Design review of the part built by this model. Coordinates are the model's own, in mm. A direction names the side the tool comes from. Give positions to 0.01 mm unless a question says otherwise; leave off trailing zeros. Order: outer loops, then holes, each group sorted by start corner. A loop starts at its lowest first (then second) coordinate and runs counter-clockwise, first axis right, second up. Notation, with made-up numbers: (56, 67.5) -> (103, 67.5) arc R22 ccw to (103, 92.5) -> close; hole circle Ø8 at (69, 79.25). An arc over 180 degrees is marked (long way). One line per item, written item: value. Start each with the question number.
1) Consider section B-B (z = 14). State the section outline as (x, y) points, plus the area to 3 significant figures.
2) Wall thickness on line 1 along X through (y, z) = (22, 13.5); line 2 along Y through (x, z) = (-5, 8.5); line 3 along Y through (x, z) = (0, 3): over which ranges is each line inside the solid? List them lowest first. Write a range as from..to.
3) The part is to be moulded in two halves that separate along X. For faces 1 (the face through (13.9, 14.8, 12.5)), 2 (the face through (11, 0, 22)), 3 (the face through (0, 26, 7)), say which applies: released by +X, released by -X, zero draft, split by the parting line, or undercut.
4) Tool access review of faces 4 (the face through (-9.6, 9.6, 18.2)), 5 (the face through (0, 11, 22)), 6 (the face through (-9.6, -9.6, 18.2)), 7 (the face through (9.015, 2.997, 11.389)), 8 (the face through (-15.5, -21.9, 12.5)): name each direction out of +Z, -Z, +X, -X, +Y, -Y from which nothing blocks a thin tool from reaching the whole face with its end or side.
5) For pin 1 (7 mm diameter, centred on x = 17.68, y = -17.68, fed in from +Z); pin 2 (8 mm diameter, centred on x = 19, z = -4.5, fed in from +Y); pin 3 (6.5 mm diameter, centred on x = -3.5, z = 23, fed in from +Y); pin 4 (3 mm diameter, centred on x = -17.5, y = -18.5, fed in from +Z), all flat-tipped, find the tip position at first contact; note any pin that passes through.
6) Consider section D-D (z = 20). State the section outline as (x, y) points, plus the area to 3 significant figures.
from build123d import *

# Parameters (mm, degrees)
F0_R            = 20
F1_DEPTH        = 17
F3_DEPTH        = 15
F4_R            = 12.5
F4_R_2          = 9.5
F5_DEPTH        = 10
F6_R            = 9.5
F7_DEPTH        = 2
F8_W            = 22
F8_H            = 22
F9_DEPTH        = 10
F10_T1_DEPTH    = 2.5403411844
F10_T3_DEPTH    = 2.5403411844
F10_T5_DEPTH    = 2.5403411844
F10_T7_DEPTH    = 2.5403411844
F10_T9_DEPTH    = 2.5403411844
F10_T11_DEPTH   = 2.5403411844
F10_T13_DEPTH   = 2.5403411844
F10_T15_DEPTH   = 2.5403411844
F10_T17_DEPTH   = 32.2867319519
F10_T19_DEPTH   = 32.2867319519
F10_T24_DEPTH   = 20.2867319519
F10_T29_DEPTH   = 20.2867319519
F10_T34_DEPTH   = 20.2867319519
F10_T39_DEPTH   = 20.2867319519
F10_T44_DEPTH   = 32.2867319519
F10_S45_R       = 9.5
F10_T46_DEPTH   = 18
F10_T50_DEPTH   = 32.2867319519
F10_S51_R       = 9.5
F10_T52_DEPTH   = 18
F10_T56_DEPTH   = 32.2867319519
F10_S57_R       = 9.5
F10_T58_DEPTH   = 18
F10_T62_DEPTH   = 32.2867319519
F10_S63_R       = 9.5
F10_T64_DEPTH   = 18
F11_R           = 10
F12_DEPTH       = 5
F13_R           = 7.5
F14_DEPTH       = 44.001
F16_D           = 5.5
F16_CBORE_D     = 9.5
F16_CBORE_DEPTH = 5


# Not quite as in the source:
# - a fillet or chamfer that OpenCascade refuses, or shapes differently, is made with other operations: its cross-section is extruded or revolved along the edge and cut away or added


with BuildPart() as f1:
    # F0 (on Top) → F1 (new body)
    with BuildSketch(Plane.XY):
        Circle(F0_R)
    extrude(amount=-F1_DEPTH)

    # F2 (on Top) → F3 (join)
    with BuildSketch(Plane.XY):
        with BuildLine():
            Line((17.7834192438, 26), (-17.7834192438, 26))
            ThreePointArc((-17.7834192438, 26), (-22.2738636074, 22.2738636074), (-26, 17.7834192438))
            Line((-26, 17.7834192438), (-26, -17.7834192438))
            ThreePointArc((-26, -17.7834192438), (-22.2738636074, -22.2738636074), (-17.7834192438, -26))
            Line((-17.7834192438, -26), (17.7834192438, -26))
            ThreePointArc((17.7834192438, -26), (22.2738636074, -22.2738636074), (26, -17.7834192438))
            Line((26, -17.7834192438), (26, 17.7834192438))
            ThreePointArc((26, 17.7834192438), (22.2738636074, 22.2738636074), (17.7834192438, 26))
        make_face()
    extrude(amount=F3_DEPTH)

    # F4 (on face) → F5 (cut)
    with BuildSketch(Plane.XY.offset(15)):
        Circle(F4_R)
        Circle(F4_R_2, mode=Mode.SUBTRACT)
    extrude(amount=-F5_DEPTH, mode=Mode.SUBTRACT)

    # F6 (on face) → F7 (join)
    with BuildSketch(Plane.XY.offset(15)):
        Circle(F6_R)
    extrude(amount=F7_DEPTH)

    # F8 (on face) → F9 (join)
    with BuildSketch(Plane.XY.offset(17)):
        Rectangle(F8_W, F8_H)
    extrude(amount=F9_DEPTH)

    # F10: chamfer of 2 on 12 edges, made by hand

    # F10_s2 → F10_t1 (cut)
    with BuildSketch(Plane(origin=(-0.3333333333, 0.3333333333, -0.3333333333), x_dir=(-0.7071067812, -0.7071067812, 0), z_dir=(-0.5773502692, 0.5773502692, -0.5773502692))):
        Polygon((-1.4142135624, 23.6784008469), (1.4142135624, 23.6784008469), (0, 21.2289111041), align=None)
    extrude(amount=F10_T1_DEPTH, mode=Mode.SUBTRACT)

    # F10_s4 → F10_t3 (cut)
    with BuildSketch(Plane(origin=(-15, 15, 15), x_dir=(-0.7071067812, -0.7071067812, 0), z_dir=(-0.5773502692, 0.5773502692, 0.5773502692))):
        Polygon((-1.4142135624, 12.2474487139), (1.4142135624, 12.2474487139), (0, 14.6969384567), align=None)
    extrude(amount=F10_T3_DEPTH, mode=Mode.SUBTRACT)

    # F10_s6 → F10_t5 (cut)
    with BuildSketch(Plane(origin=(0.3333333333, 0.3333333333, -0.3333333333), x_dir=(-0.7071067812, 0.7071067812, 0), z_dir=(0.5773502692, 0.5773502692, -0.5773502692))):
        Polygon((1.4142135624, 23.6784008469), (-1.4142135624, 23.6784008469), (0, 21.2289111041), align=None)
    extrude(amount=F10_T5_DEPTH, mode=Mode.SUBTRACT)

    # F10_s8 → F10_t7 (cut)
    with BuildSketch(Plane(origin=(15, 15, 15), x_dir=(-0.7071067812, 0.7071067812, 0), z_dir=(0.5773502692, 0.5773502692, 0.5773502692))):
        Polygon((1.4142135624, 12.2474487139), (-1.4142135624, 12.2474487139), (0, 14.6969384567), align=None)
    extrude(amount=F10_T7_DEPTH, mode=Mode.SUBTRACT)

    # F10_s10 → F10_t9 (cut)
    with BuildSketch(Plane(origin=(0.3333333333, -0.3333333333, -0.3333333333), x_dir=(0.7071067812, 0.7071067812, 0), z_dir=(0.5773502692, -0.5773502692, -0.5773502692))):
        Polygon((1.4142135624, 23.6784008469), (0, 21.2289111041), (-1.4142135624, 23.6784008469), align=None)
    extrude(amount=F10_T9_DEPTH, mode=Mode.SUBTRACT)

    # F10_s12 → F10_t11 (cut)
    with BuildSketch(Plane(origin=(15, -15, 15), x_dir=(0.7071067812, 0.7071067812, 0), z_dir=(0.5773502692, -0.5773502692, 0.5773502692))):
        Polygon((1.4142135624, 12.2474487139), (0, 14.6969384567), (-1.4142135624, 12.2474487139), align=None)
    extrude(amount=F10_T11_DEPTH, mode=Mode.SUBTRACT)

    # F10_s14 → F10_t13 (cut)
    with BuildSketch(Plane(origin=(-0.3333333333, -0.3333333333, -0.3333333333), x_dir=(0.7071067812, -0.7071067812, 0), z_dir=(-0.5773502692, -0.5773502692, -0.5773502692))):
        Polygon((-1.4142135624, 23.6784008469), (0, 21.2289111041), (1.4142135624, 23.6784008469), align=None)
    extrude(amount=F10_T13_DEPTH, mode=Mode.SUBTRACT)

    # F10_s16 → F10_t15 (cut)
    with BuildSketch(Plane(origin=(-15, -15, 15), x_dir=(0.7071067812, -0.7071067812, 0), z_dir=(-0.5773502692, -0.5773502692, 0.5773502692))):
        Polygon((-1.4142135624, 12.2474487139), (0, 14.6969384567), (1.4142135624, 12.2474487139), align=None)
    extrude(amount=F10_T15_DEPTH, mode=Mode.SUBTRACT)

    # F10_s18 → F10_t17 (cut)
    with BuildSketch(Plane.XZ.offset(-16.1433659759)):
        Polygon((-11, 25), (-9, 27), (-11, 27), align=None)
        Polygon((11, 25), (9, 27), (11, 27), align=None)
    extrude(amount=F10_T17_DEPTH, mode=Mode.SUBTRACT)

    # F10_s20 → F10_t19 (cut)
    with BuildSketch(Plane.YZ.offset(-16.1433659759)):
        Polygon((-9, 27), (-11, 25), (-11, 27), align=None)
        Polygon((11, 25), (9, 27), (11, 27), align=None)
    extrude(amount=F10_T19_DEPTH, mode=Mode.SUBTRACT)


with BuildPart() as f10_tool22:
    # F10_s23 → F10_t24 (new body)
    with BuildSketch(Plane.XY.offset(11.8566340241)):
        Polygon((-9, 11), (-11, 9), (-11, 11), align=None)
    extrude(amount=F10_T24_DEPTH)

    split(bisect_by=Plane.XY.offset(15), keep=Keep.TOP)


with BuildPart() as f1_1:
    add(f1.part)

    # F10_t21: cut F10_tool22
    add(f10_tool22.part, mode=Mode.SUBTRACT)


with BuildPart() as f10_tool27:
    # F10_s28 → F10_t29 (new body)
    with BuildSketch(Plane.XY.offset(11.8566340241)):
        Polygon((9, 11), (11, 9), (11, 11), align=None)
    extrude(amount=F10_T29_DEPTH)

    split(bisect_by=Plane.XY.offset(15), keep=Keep.TOP)


with BuildPart() as f1_2:
    add(f1_1.part)

    # F10_t26: cut F10_tool27
    add(f10_tool27.part, mode=Mode.SUBTRACT)


with BuildPart() as f10_tool32:
    # F10_s33 → F10_t34 (new body)
    with BuildSketch(Plane.XY.offset(11.8566340241)):
        Polygon((11, -9), (9, -11), (11, -11), align=None)
    extrude(amount=F10_T34_DEPTH)

    split(bisect_by=Plane.XY.offset(15), keep=Keep.TOP)


with BuildPart() as f1_3:
    add(f1_2.part)

    # F10_t31: cut F10_tool32
    add(f10_tool32.part, mode=Mode.SUBTRACT)


with BuildPart() as f10_tool37:
    # F10_s38 → F10_t39 (new body)
    with BuildSketch(Plane.XY.offset(11.8566340241)):
        Polygon((-11, -9), (-9, -11), (-11, -11), align=None)
    extrude(amount=F10_T39_DEPTH)

    split(bisect_by=Plane.XY.offset(15), keep=Keep.TOP)


with BuildPart() as f1_4:
    add(f1_3.part)

    # F10_t36: cut F10_tool37
    add(f10_tool37.part, mode=Mode.SUBTRACT)


with BuildPart() as f10_tool42:
    # F10_s43 → F10_t44 (new body)
    with BuildSketch(Plane.XZ.offset(-16.1433659759)):
        Polygon((-11, 19), (-9, 17), (-11, 17), align=None)
    extrude(amount=F10_T44_DEPTH)

    # F10_s45 → F10_t46 (cut, symmetric)
    with BuildSketch(Plane.XY.offset(18)):
        Circle(F10_S45_R)
    extrude(amount=F10_T46_DEPTH, both=True, mode=Mode.SUBTRACT)


with BuildPart() as f1_5:
    add(f1_4.part)

    # F10_t41: cut F10_tool42
    add(f10_tool42.part, mode=Mode.SUBTRACT)


with BuildPart() as f10_tool48:
    # F10_s49 → F10_t50 (new body)
    with BuildSketch(Plane.XZ.offset(16.1433659759)):
        Polygon((11, 19), (9, 17), (11, 17), align=None)
    extrude(amount=-F10_T50_DEPTH)

    # F10_s51 → F10_t52 (cut, symmetric)
    with BuildSketch(Plane.XY.offset(18)):
        Circle(F10_S51_R)
    extrude(amount=F10_T52_DEPTH, both=True, mode=Mode.SUBTRACT)


with BuildPart() as f1_6:
    add(f1_5.part)

    # F10_t47: cut F10_tool48
    add(f10_tool48.part, mode=Mode.SUBTRACT)


with BuildPart() as f10_tool54:
    # F10_s55 → F10_t56 (new body)
    with BuildSketch(Plane.YZ.offset(-16.1433659759)):
        Polygon((-9, 17), (-11, 19), (-11, 17), align=None)
    extrude(amount=F10_T56_DEPTH)

    # F10_s57 → F10_t58 (cut, symmetric)
    with BuildSketch(Plane.XY.offset(18)):
        Circle(F10_S57_R)
    extrude(amount=F10_T58_DEPTH, both=True, mode=Mode.SUBTRACT)


with BuildPart() as f1_7:
    add(f1_6.part)

    # F10_t53: cut F10_tool54
    add(f10_tool54.part, mode=Mode.SUBTRACT)


with BuildPart() as f10_tool60:
    # F10_s61 → F10_t62 (new body)
    with BuildSketch(Plane.YZ.offset(16.1433659759)):
        Polygon((11, 19), (9, 17), (11, 17), align=None)
    extrude(amount=-F10_T62_DEPTH)

    # F10_s63 → F10_t64 (cut, symmetric)
    with BuildSketch(Plane.XY.offset(18)):
        Circle(F10_S63_R)
    extrude(amount=F10_T64_DEPTH, both=True, mode=Mode.SUBTRACT)


with BuildPart() as f1_8:
    add(f1_7.part)

    # F10_t59: cut F10_tool60
    add(f10_tool60.part, mode=Mode.SUBTRACT)

    # F11 (on face) → F12 (cut)
    with BuildSketch(Plane(origin=(0, 0, -17), x_dir=(1, 0, 0), z_dir=(0, 0, -1))):
        Circle(F11_R)
    extrude(amount=-F12_DEPTH, mode=Mode.SUBTRACT)

    # F13 (on face) → F14 (cut, through all)
    with BuildSketch(Plane.XY.offset(27)):
        Circle(F13_R)
    extrude(amount=-F14_DEPTH, mode=Mode.SUBTRACT)

    # F16 (through all)
    with Locations(Plane.XY.offset(15)):
        with Locations((17.6776695297, 17.6776695297), (17.6776695297, -17.6776695297), (-17.6776695297, -17.6776695297), (-17.6776695297, 17.6776695297)):
            CounterBoreHole(F16_D / 2, F16_CBORE_D / 2, F16_CBORE_DEPTH)


solid = f1_8.part
Checked values:
1. outline: (-26, -17.78) arc R31.5 ccw to (-17.78, -26) -> (17.78, -26) arc R31.5 ccw to (26, -17.78) -> (26, 17.78) arc R31.5 ccw to (17.78, 26) -> (-17.78, 26) arc R31.5 ccw to (-26, 17.78) -> close; circle Ø19 at (0, 0); hole circle Ø9.5 at (-17.68, -17.68); hole circle Ø9.5 at (-17.68, 17.68); hole circle Ø25 at (0, 0); hole circle Ø15 at (0, 0); hole circle Ø9.5 at (17.68, -17.68); hole circle Ø9.5 at (17.68, 17.68)
1. area: 1,920 mm^2
2. line 1: x = -22.54..-19.65, -15.71..15.71, 19.65..22.54
2. line 2: y = -26..-11.46, -8.08..-5.59, 5.59..8.08, 11.46..26
2. line 3: y = -26..-7.5, 7.5..26
3. face 1: undercut
3. face 2: released by +X
3. face 3: zero draft
4. face 4: -X, +Y
4. face 5: +Z, +X, -X, +Y
4. face 6: -X, -Y
4. face 7: none
4. face 8: +Z
5. pin 1: stops at z = 10
5. pin 2: stops at y = 13.23
5. pin 3: stops at y = 11
5. pin 4: passes through
6. outline: (-11, -9) -> (-9, -11) -> (9, -11) -> (11, -9) -> (11, 9) -> (9, 11) -> (-9, 11) -> (-11, 9) -> close; hole circle Ø15 at (0, 0)
6. area: 299 mm^2
